from build123d import *

# Parameters (mm, degrees)
BOSS_EXTRU_1_DEPTH      = 430
BOSS_EXTRU_2_DEPTH      = 250
BOSS_EXTRU_3_DEPTH      = 680
ESQUISSE2_W             = 200
ESQUISSE2_H             = 250
ENL_V_MAT_EXTRU_2_DEPTH = 680
ESQUISSE3_W             = 70
ESQUISSE3_H             = 70
ENL_V_MAT_EXTRU_3_DEPTH = 100
ESQUISSE4_W             = 70
ESQUISSE4_H             = 70
ENL_V_MAT_EXTRU_4_DEPTH = 100


with BuildPart() as part:
    # Esquisse1 → Boss.-Extru.1 (new body)
    with BuildSketch(Plane(origin=(0, 0, 0), x_dir=(0, 0, -1), z_dir=(1, 0, 0))):
        with BuildLine():
            ThreePointArc((292.5, 0), (-50.590265862, 288.09178225), (-275, -99.65565714))
            Line((-275, -99.65565714), (-8.291561976, -99.65565714))
            ThreePointArc((-8.291561976, -99.65565714), (-67.715743378, 73.583816827), (100, 0))
            ThreePointArc((100, 0), (73.583816827, -67.715743378), (8.291561976, -99.65565714))
            Line((8.291561976, -99.65565714), (275, -99.65565714))
            ThreePointArc((275, -99.65565714), (288.09178225, -50.590265862), (292.5, 0))
        make_face()
        with BuildLine():
            Line((-8.291561976, -99.65565714), (-275, -99.65565714))
            ThreePointArc((-275, -99.65565714), (0, -292.5), (275, -99.65565714))
            Line((275, -99.65565714), (8.291561976, -99.65565714))
            ThreePointArc((8.291561976, -99.65565714), (0, -100), (-8.291561976, -99.65565714))
        make_face()
        with BuildLine():
            ThreePointArc((275, -99.65565714), (0, -292.5), (-275, -99.65565714))
            Line((-275, -99.65565714), (-100, -1224.65565714))
            Line((-100, -1224.65565714), (100, -1224.65565714))
            Line((100, -1224.65565714), (275, -99.65565714))
        make_face()
        with BuildLine():
            Line((100, -1224.65565714), (-100, -1224.65565714))
            Line((-100, -1224.65565714), (-80.555555556, -1349.65565714))
            Line((-80.555555556, -1349.65565714), (-80, -1349.65565714))
            ThreePointArc((-80, -1349.65565714), (0, -1269.65565714), (80, -1349.65565714))
            Line((80, -1349.65565714), (80.555555556, -1349.65565714))
            Line((80.555555556, -1349.65565714), (100, -1224.65565714))
        make_face()
        with BuildLine():
            Line((-80.555555556, -1349.65565714), (-100, -1224.65565714))
            Line((-100, -1224.65565714), (-100, -1399.65565714))
            ThreePointArc((-100, -1399.65565714), (-78.033008589, -1452.688665729), (-25, -1474.65565714))
            Line((-25, -1474.65565714), (25, -1474.65565714))
            ThreePointArc((25, -1474.65565714), (78.033008589, -1452.688665729), (100, -1399.65565714))
            Line((100, -1399.65565714), (100, -1224.65565714))
            Line((100, -1224.65565714), (80.555555556, -1349.65565714))
            Line((80.555555556, -1349.65565714), (80, -1349.65565714))
            ThreePointArc((80, -1349.65565714), (0, -1429.65565714), (-80, -1349.65565714))
            Line((-80, -1349.65565714), (-80.555555556, -1349.65565714))
        make_face()
    extrude(amount=BOSS_EXTRU_1_DEPTH)



with BuildPart() as body_2:
    # Esquisse1_3 → Boss.-Extru.2 (new body)
    with BuildSketch(Plane(origin=(0, 0, 0), x_dir=(0, 0, -1), z_dir=(1, 0, 0))):
        with BuildLine():
            ThreePointArc((80, -1349.65565714), (0, -1269.65565714), (-80, -1349.65565714))
            Line((-80, -1349.65565714), (80, -1349.65565714))
        make_face()
        with BuildLine():
            Line((80, -1349.65565714), (-80, -1349.65565714))
            ThreePointArc((-80, -1349.65565714), (0, -1429.65565714), (80, -1349.65565714))
        make_face()
    extrude(amount=-BOSS_EXTRU_2_DEPTH)


with BuildPart() as part_1:
    add(part.part)

    add(body_2.part)  # Boss.-Extru.3 merges body 2
    # Esquisse1_5 → Boss.-Extru.3 (add)
    with BuildSketch(Plane(origin=(0, 0, 0), x_dir=(0, 0, -1), z_dir=(1, 0, 0))):
        with BuildLine():
            ThreePointArc((80, -1349.65565714), (0, -1269.65565714), (-80, -1349.65565714))
            Line((-80, -1349.65565714), (80, -1349.65565714))
        make_face()
        with BuildLine():
            Line((80, -1349.65565714), (-80, -1349.65565714))
            ThreePointArc((-80, -1349.65565714), (0, -1429.65565714), (80, -1349.65565714))
        make_face()
    extrude(amount=BOSS_EXTRU_3_DEPTH)

    # Esquisse2 → Enl_v. mat.-Extru.2 (cut)
    with BuildSketch(Plane.XY.offset(100)):
        with Locations((215, -1349.65565714)):
            Rectangle(ESQUISSE2_W, ESQUISSE2_H)
    extrude(amount=-ENL_V_MAT_EXTRU_2_DEPTH, mode=Mode.SUBTRACT)

    # Esquisse3 → Enl_v. mat.-Extru.3 (cut)
    with BuildSketch(Plane.ZY.offset(250)):
        with Locations((0, -1349.65565714)):
            Rectangle(ESQUISSE3_W, ESQUISSE3_H)
    extrude(amount=-ENL_V_MAT_EXTRU_3_DEPTH, mode=Mode.SUBTRACT)

    # Esquisse4 → Enl_v. mat.-Extru.4 (cut)
    with BuildSketch(Plane(origin=(680, 0, 0), x_dir=(0, 0, -1), z_dir=(1, 0, 0))):
        with Locations((0, -1349.65565714)):
            Rectangle(ESQUISSE4_W, ESQUISSE4_H)
    extrude(amount=-ENL_V_MAT_EXTRU_4_DEPTH, mode=Mode.SUBTRACT)


solid = part_1.part
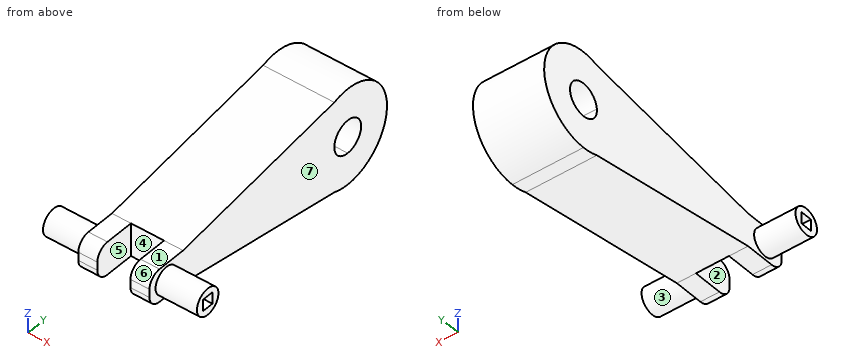
Input: part model. Units: mm. Frame: model coordinates. Face numbers are marked on the shaded views. A direction names the side the tool comes from. Give positions to 0.01 mm unless a question says otherwise; leave off trailing zeros. Loops run counter-clockwise (first coordinate to the right, second up) from the corner with the lowest first, then second, coordinate; pieces in that order, holes last. Notation, with made-up numbers: M -6,-34 L 33,-34 A19 ccw 33,3 Z; hole C -25.5,85.5 d3. An arc over 180 degrees is marked long. Use one line per item in the form item = value.
1. Section query C-C, the plane z = 209.5. Return the cut outline in (x, y), and give its area (3 significant figures).
Numbers:
outline = M 0,-520.73 L 430,-520.73 L 430,204.12 L 0,204.12 Z
area = 312,000 mm²
2. Section query A-A, the plane x = 408. Return the cut outline in (y, z).
Numbers:
outline = M -1474.66,-25 A75 ccw -1399.66,-100 L -1224.66,-100 L -99.66,-275 A292.5 ccw long -99.66,275 L -1224.66,100 L -1399.66,100 A75 ccw -1474.66,25 Z; hole C 0,0 d200
3. Section query D-D, the plane x = -120.5. Return the cut outline in (y, z), and give its area (3 significant figures).
Numbers:
outline = C -1349.66,0 d160
area = 20,100 mm²
4. Line query: L1, parallel to Y at x = 277.5, z = 0; L2, parallel to X at y = -1231, z = -70.5; L3, parallel to Z at x = 9.5, y = 2. Output: solid intervals per line, ascending.
Numbers:
L1 = -1224.66 to -100, 100 to 292.5
L2 = 0 to 115, 315 to 430
L3 = -292.49 to -99.98, 99.98 to 292.49
5. Reachability of the marked faces 1, 2 and 3 from +Z, -Z, +X, -X, +Y, -Y: full face, straight path, thin tool, end or side. Return the list, or none.
Numbers:
face_1 = +Z, +X, -X, -Y
face_2 = +Z, -Z, -Y
face_3 = +X
6. First-contact query: pin 1 (21 mm diameter, centred on x = 643, z = 15, fed in from +Y); pin 2 (5 mm diameter, centred on y = -374.5, z = -75.5, fed in from +X); pin 3 (1.5 mm diameter, centred on x = 131, z = -81.5, fed in from +Y). Flat tips, straight axial feed; report the tip coordinate or a pass-through.
Numbers:
pin_1 = -1269.78
pin_2 = 430
pin_3 = 281.13
7. Pull-direction query (X, two-part tool) for the marked faces 4, 5, 6 and 7; classes: released by +X, released by -X, zero draft, split by the parting line, or undercut.
Numbers:
face_4 = undercut
face_5 = undercut
face_6 = zero draft
face_7 = released by +X
8. Section query B-B, the plane y = -21.5. Return the cut outline in (x, z), and give its area (3 significant figures).
Numbers:
outline = M 0,-291.71 L 430,-291.71 L 430,-97.66 L 0,-97.66 Z; M 0,97.66 L 430,97.66 L 430,291.71 L 0,291.71 Z
area = 167,000 mm²
